Here's how the part is built. I have some questions about the finished solid (model axes, mm). A direction names the side the tool comes from. Give positions to 0.01 mm unless a question says otherwise; leave off trailing zeros. Loops run counter-clockwise (first coordinate to the right, second up) from the corner with the lowest first, then second, coordinate; pieces in that order, holes last. Notation, with made-up numbers: (42.5, 17.25) -> (53.5, 17.25) arc R25 ccw to (53.5, 37.25) -> close; hole circle Ø11 at (9.5, 60.5). An arc over 180 degrees is marked (long way). Answer in a Markdown table with one row per item. Add a question column.
Item 1: If we section it at D-D (y = 51): Write out the boundary of the cut face in (x, z) (3 decimals), then the cut area to 3 significant figures.
Item 2: We'd pull the mould along X, two halves only. Please class faces 1 (the face through (0, -6.35, 22)), 2 (the face through (22.225, 29, 22)), 3 (the face through (35.8, 49.65, 21.91)): released by +X, released by -X, zero draft, split by the parting line, or undercut.
Item 3: If I drill on line 1 (X direction, y = 9, z = 23) (3 decimals); line 2 (Y direction, x = -2, z = 20); line 3 (Y direction, x = 71, z = 21), over which ranges is the centre line in solid material (lowest first)?
Item 4: If we section it at B-B (z = 33): Write out the boundary of the cut face in (x, y) (3 decimals), then the cut area to 3 significant figures.
Item 5: Which directions (+Z, -Z, +X, -X, +Y, -Y) give clear straight access to the entire face, cutting with the end or side of a thin tool? Please do faces 4 (the face through (-57, 57.937, 22)), 5 (the face through (68, 56.667, 22)), 6 (the face through (0, 0, 22)), 7 (the face through (-28.575, 18, 22)).
Item 6: If we section it at C-C (x = 14): Write out the boundary of the cut face in (y, z), then the cut area to 3 significant figures.
Item 7: For P1, Ø1, axis at x = -45.5, z = 11, coming from the -Y side; P2, Ø13.5, axis at y = 31.5, z = 27.5, coming from the +X side (3 decimals); P3, Ø22, axis at y = 41, z = 30.5, coming from the -X side; P4, Ø4.5, axis at x = -83.185, z = 22.225, coming from the -Y side, each with a flat end and sliding along its axis, tell me the tip position at first contact or that it passes through.
Item 8: If we section it at A-A (y = 4): Write out the boundary of the cut face in (x, z) (3 decimals), then the cut area to 3 significant figures.
```python
from build123d import *

# Parameters (mm, degrees)
BOSS_EXTRUDE1_DEPTH = 44.45
SKETCH2_R           = 3.937
CUT_EXTRUDE1_DEPTH  = 121.103292327


with BuildPart() as part:
    # Sketch1 → Boss-Extrude1 (new body)
    with BuildSketch(Plane.XY):
        Polygon((-22.225, 0), (22.225, 0), (22.225, 57.9374), (28.575, 57.9374), (92.075, 57.9374), (92.075, 56.6674), (42.818141465, 56.6674), (28.575, 42.424258535), (28.575, -6.35), (-28.575, -6.35), (-28.575, 42.424258535), (-42.818141465, 56.6674), (-92.075, 56.6674), (-92.075, 57.9374), (-28.575, 57.9374), (-22.225, 57.9374), align=None)
    extrude(amount=BOSS_EXTRUDE1_DEPTH)

    # Sketch2 → Cut-Extrude1 (cut, through all)
    with BuildSketch(Plane.XZ.offset(-56.6674)):
        with Locations((83.185, 22.225)):
            Circle(SKETCH2_R)
        with Locations(Location((-83.185, 22.225, 0), (0, 0, 180))):
            Circle(SKETCH2_R)
    extrude(amount=-CUT_EXTRUDE1_DEPTH, mode=Mode.SUBTRACT)


solid = part.part
```
Recorded:
| question | item | result |
|---|---|---|
| 1 | outline | (-37.151, 0) -> (-22.225, 0) -> (-22.225, 44.45) -> (-37.151, 44.45) -> close; (22.225, 0) -> (37.151, 0) -> (37.151, 44.45) -> (22.225, 44.45) -> close |
| 1 | area | 1,330 mm^2 |
| 2 | face 1 | zero draft |
| 2 | face 2 | undercut |
| 2 | face 3 | released by +X |
| 3 | line 1 | x = -28.575 to -22.225, 22.225 to 28.575 |
| 3 | line 2 | y = -6.35 to 0 |
| 3 | line 3 | y = 56.67 to 57.94 |
| 4 | outline | (-92.075, 56.667) -> (-42.818, 56.667) -> (-28.575, 42.424) -> (-28.575, -6.35) -> (28.575, -6.35) -> (28.575, 42.424) -> (42.818, 56.667) -> (92.075, 56.667) -> (92.075, 57.937) -> (22.225, 57.937) -> (22.225, 0) -> (-22.225, 0) -> (-22.225, 57.937) -> (-92.075, 57.937) -> close |
| 4 | area | 1,460 mm^2 |
| 5 | face 4 | +Z, -Z, +X, -X, +Y |
| 5 | face 5 | +Z, -Z, +X, -Y |
| 5 | face 6 | +Z, -Z, +Y |
| 5 | face 7 | +Z, -Z, -X, -Y |
| 6 | outline | (-6.35, 0) -> (0, 0) -> (0, 44.45) -> (-6.35, 44.45) -> close |
| 6 | area | 282 mm^2 |
| 7 | P1 | stops at y = 56.67 |
| 7 | P2 | stops at x = 28.575 |
| 7 | P3 | stops at x = -38.15 |
| 7 | P4 | passes through |
| 8 | outline | (-28.575, 0) -> (-22.225, 0) -> (-22.225, 44.45) -> (-28.575, 44.45) -> close; (22.225, 0) -> (28.575, 0) -> (28.575, 44.45) -> (22.225, 44.45) -> close |
| 8 | area | 565 mm^2 |
